Here's how the part is built. I have some questions about the finished solid (model axes, mm). Give positions to 0.01 mm unless a question says otherwise; leave off trailing zeros. Loops run counter-clockwise (first coordinate to the right, second up) from the corner with the lowest first, then second, coordinate; pieces in that order, holes last.
Q1. I need wall thicknesses on probe 1 along X at (y, z) = (-1, 114.5); probe 2 along Z at (x, y) = (-51, 0.5); probe 3 along X at (y, z) = (-7, -231). Which ranges of each line are inside material? Lowest first, please.
Q2. Suppose I cut it at A-A (y = -17). List the corners of the cut face in (x, z) for me.
Q3. I'm going to push flat-ended pins straight in: P1, Ø6, axis at y = -11.5, z = 135, coming from the +X side; P2, Ø15, axis at y = -5, z = 32.5, coming from the -X side; P3, Ø8, axis at x = 77, y = -1, coming from the +Z side. Where does each tip first touch, or does it pass through?
Q4. Suppose I cut it at B-B (z = 29.5). List the corners of the cut face in (x, y) for me.
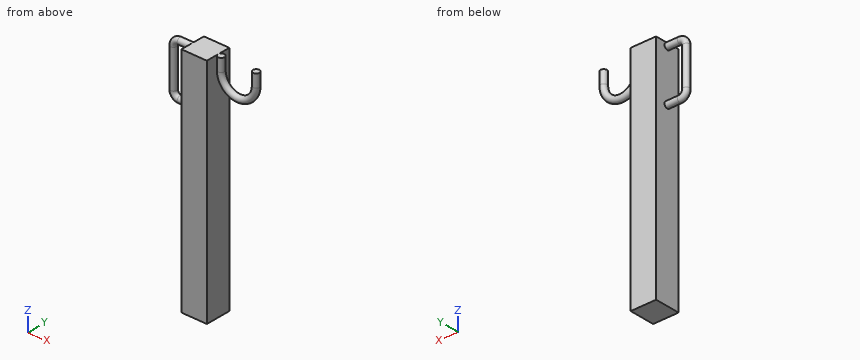
```python
from build123d import *

# Parameters (mm, degrees)
F0_W          = 50.8
F0_H          = 50.8
F1_DEPTH      = 203.2
F1_DEPTH_BACK = 254
F3_R          = 6.604
F6_R          = 6.35


with BuildPart() as f1:
    # F0 (on Top) → F1 (new body, two sides)
    with BuildSketch(Plane.XY) as f1_sk:
        Rectangle(F0_W, F0_H)
    extrude(amount=F1_DEPTH)
    extrude(f1_sk.sketch, amount=-F1_DEPTH_BACK)

    # F4: sweep along a path in F2
    with BuildLine(Plane.XZ) as f4_path:
        Line((101.6, 203.2), (101.6, 177.8))
        ThreePointArc((101.6, 177.8), (66.675, 142.875), (31.75, 177.8))
        Line((31.75, 177.8), (31.75, 203.2))
    # F3 (on face) → F4 (sweep)
    with BuildSketch(Plane.XY.offset(203.2)):
        with Locations((31.75, 0)):
            Circle(F3_R)
    sweep(path=f4_path.line)

    # F7: sweep along a path in F5
    with BuildLine(Plane.XZ) as f7_path:
        Line((-25.4, 196.85), (-50.8, 196.85))
        ThreePointArc((-50.8, 196.85), (-59.7802561211, 193.1302561211), (-63.5, 184.15))
        Line((-63.5, 184.15), (-63.5, 107.95))
        ThreePointArc((-63.5, 107.95), (-59.7802561211, 98.9697438789), (-50.8, 95.25))
        Line((-50.8, 95.25), (-25.3296792507, 95.25))
    # F6 (on face) → F7 (sweep)
    with BuildSketch(Plane(origin=(-25.4, 0, 0), x_dir=(0, -1, 0), z_dir=(-1, 0, 0))):
        with Locations((0, 196.85)):
            Circle(F6_R)
    sweep(path=f7_path.line)


solid = f1.part
```
Solutions:
1. probe 1: x = -69.77 to -57.23, -25.4 to 25.4
1. probe 2: z = 88.92 to 101.58, 190.52 to 203.18
1. probe 3: x = -25.4 to 25.4
2. outline: (-25.4, -254) - (25.4, -254) - (25.4, 203.2) - (-25.4, 203.2) - close
3. P1: stops at x = 25.4
3. P2: stops at x = -25.4
3. P3: stops at z = 153.33
4. outline: (-25.4, -25.4) - (25.4, -25.4) - (25.4, 25.4) - (-25.4, 25.4) - close
